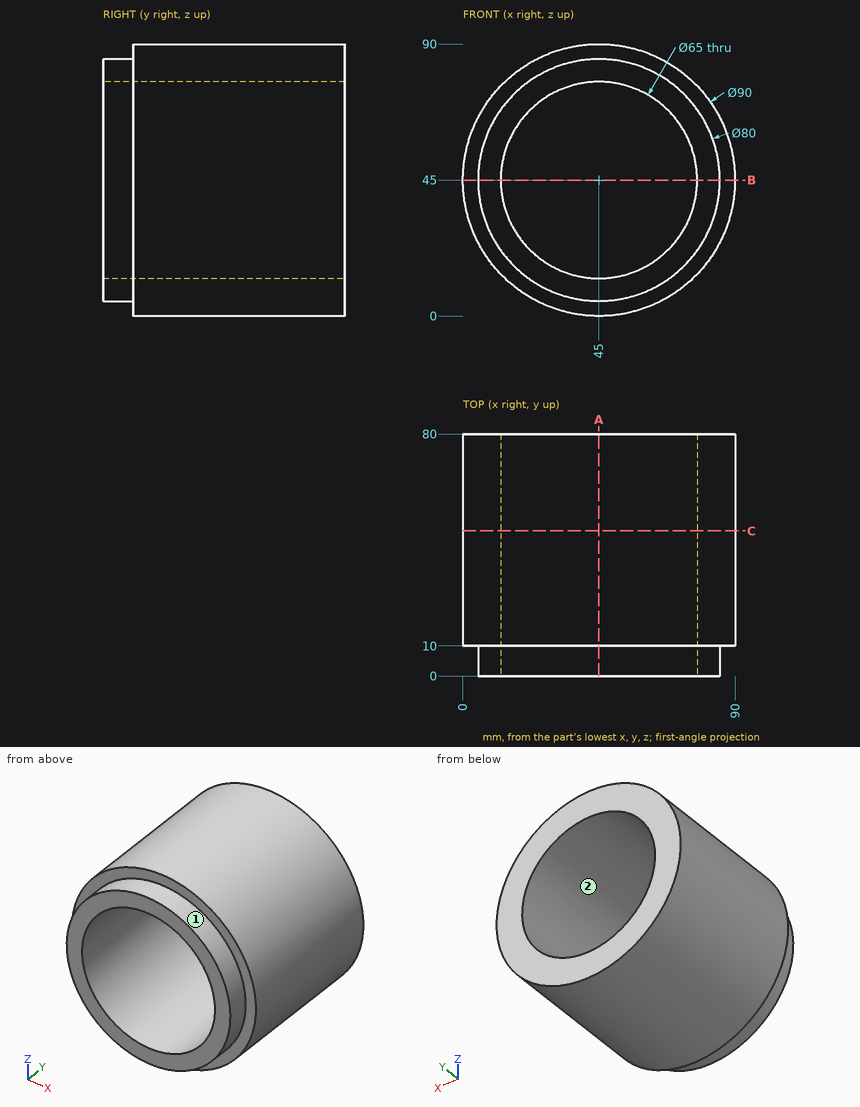
Here's the drawing with two shaded views (mm, measured from the low corner). I have some questions. A direction names the side the tool comes from. Round coordinates to 2 decimals unless told otherwise and drop trailing zeros. Loops run counter-clockwise (first coordinate to the right, second up) from the corner with the lowest first, then second, coordinate; pieces in that order, holes last. Notation, with made-up numbers: (89.25, -5.75) - (138.25, -5.75) arc R31 cw to (138.25, 27.25) - close; hole circle Ø6 at (-28, 12). An arc over 180 degrees is marked (long way). Use CSV: the item, a comma, the result in double quotes. Start each with the question number.
1) If we section it at A-A on x = 45: Write out the boundary of the cut face in (y, z), plus the area to 3 significant figures.
2) For pin 1 Ø5 at (x, y) = (63.5, 36.5) entering from +Z; pin 2 Ø5 at (y, z) = (67.5, 16) entering from +X; pin 3 Ø4 at (x, y) = (10.5, 22.5) entering from -Z, each with a flat end and sliding along its axis, tell me the tip position at first contact or that it passes through.
3) If we section it at C-C on y = 48: Write out the boundary of the cut face in (x, z).
4) Please list where these lines run through material, in increasing order: probe 1 along X at (y, z) = (56, 45); probe 2 along Z at (x, y) = (46, 74.5); probe 3 along Z at (x, y) = (56, 63.5). Write a range as [from, to].
5) If we section it at B-B on z = 45: Write out the boundary of the cut face in (x, y), plus the area to 3 significant figures.
6) For the marked faces 1 and 2, which set-ups out of +Z, -Z, +X, -X, +Y, -Y let a thin tool reach every point of the face, with its end or its side?
Geometry results:
1,outline,"(0, 5) - (10, 5) - (10, 0) - (80, 0) - (80, 12.5) - (0, 12.5) - close; (0, 77.5) - (80, 77.5) - (80, 90) - (10, 90) - (10, 85) - (0, 85) - close"
1,area,"1,900 mm2"
2,pin 1,"stops at z = 87.06"
2,pin 2,"stops at x = 81.37"
2,pin 3,"stops at z = 13.88"
3,outline,"circle Ø90 at (45, 45); hole circle Ø65 at (45, 45)"
4,probe 1,"x = [0, 12.5], [77.5, 90]"
4,probe 2,"z = [0.01, 12.52], [77.48, 89.99]"
4,probe 3,"z = [1.37, 14.42], [75.58, 88.63]"
5,outline,"(0, 10) - (5, 10) - (5, 0) - (12.5, 0) - (12.5, 80) - (0, 80) - close; (77.5, 0) - (85, 0) - (85, 10) - (90, 10) - (90, 80) - (77.5, 80) - close"
5,area,"1,900 mm2"
6,face 1,"-Y"
6,face 2,"+Y, -Y"
